Check sheet for the modelled part. Datum: model origin and axes. Units: mm. A direction names the side the tool comes from. Round coordinates to 2 decimals unless told otherwise and drop trailing zeros. Write each loop counter-clockwise with the first axis right and the second up, starting at its lowest first coordinate (ties: lowest second). Pieces come first, ordered by that corner, then holes. Notation, with made-up numbers: (-23.5, 10.25) -> (-2.5, 10.25) arc R27 ccw to (-2.5, 32.25) -> close; hole circle Ø11 at (53, 35). An arc over 180 degrees is marked (long way). Put each result on its own line as item: value. Start each with the question number.
from build123d import *

# Parameters (mm, degrees)
F0_R     = 19.05
F0_R_2   = 16.51
F0_R_3   = 7.62
F0_R_4   = 4.8407005088
F1_DEPTH = 5
F2_START = 5
F0_R_5   = 2.25
F2_DEPTH = 10
F3_START = 12
F3_DEPTH = 8


with BuildPart() as f1:
    # F0 (on Top) → F1 (new body)
    with BuildSketch(Plane.XY):
        Circle(F0_R)
        Circle(F0_R_2, mode=Mode.SUBTRACT)
        Circle(F0_R_2)
        Circle(F0_R_3, mode=Mode.SUBTRACT)
        Circle(F0_R_3)
        Circle(F0_R_4, mode=Mode.SUBTRACT)
    extrude(amount=F1_DEPTH)

    # F0 (on Top) → F2 (join)
    with BuildSketch(Plane.XY.offset(F2_START)):
        Circle(F0_R)
        Circle(F0_R_2, mode=Mode.SUBTRACT)
        Circle(F0_R_3)
        Circle(F0_R_4, mode=Mode.SUBTRACT)
        Circle(F0_R_4)
        Polygon((-2.865183893, 3.6227137055), (1.7047701531, 4.2926788907), (4.5699540462, 0.6699651851), (2.865183893, -3.6227137055), (-1.7047701531, -4.2926788907), (-4.5699540462, -0.6699651851), align=None, mode=Mode.SUBTRACT)
        Polygon((4.5699540462, 0.6699651851), (1.7047701531, 4.2926788907), (-2.865183893, 3.6227137055), (-4.5699540462, -0.6699651851), (-1.7047701531, -4.2926788907), (2.865183893, -3.6227137055), align=None)
        Circle(F0_R_5, mode=Mode.SUBTRACT)
    extrude(amount=F2_DEPTH)

    # F0 (on Top) → F3 (cut)
    with BuildSketch(Plane.XY.offset(F3_START)):
        Polygon((4.5699540462, 0.6699651851), (1.7047701531, 4.2926788907), (-2.865183893, 3.6227137055), (-4.5699540462, -0.6699651851), (-1.7047701531, -4.2926788907), (2.865183893, -3.6227137055), align=None)
        Circle(F0_R_5, mode=Mode.SUBTRACT)
    extrude(amount=F3_DEPTH, mode=Mode.SUBTRACT)


solid = f1.part
1. Section check A-A, the plane z = 13.25. Enter the section's corners in (x, y).
2. Material ranges on L1, parallel to Y at x = 0, z = 10; L2, parallel to X at y = 5, z = 9.75; L3, parallel to X at y = -4.5, z = 9.25, recorded low to high. Write a range as [from, to].
3. Section check D-D, the plane z = 6.75. Enter the section's corners in (x, y).
4. Section check C-C, the plane x = 0. Enter the section's corners in (y, z).
5. Gauge pin test, flat ends, axial feed: P1, Ø4.5, axis at x = -1.5, y = 0, coming from the +Z side; P2, Ø6, axis at x = 0, y = 0, coming from the -Z side; P3, Ø1, axis at x = 0.5, y = -9.5, coming from the +Z side. Record the tip position at first contact, or that the pin passes through.
6. Draft check along Y on faces 1 (the cylindrical face through (-15.12, -11.59, 7.4)), 2 (the flat face through (-6, 16, 15)), 3 (the flat face through (-0.548, 3.962, 13.479)), 4 (the cylindrical face through (4.62, 1.45, 2.46)). Enter one of: released by +Y, released by -Y, zero draft, split by the parting line, or undercut.
7. Section check B-B, the plane y = 14. Enter the section's corners in (x, z), then the cut area to 3 significant figures.
8. Access from +Z, -Z, +X, -X, +Y, -Y to the whole of each face (thin tool, end or side, straight path). Record for faces 5 (the flat face through (3.3, -3.3, 15)), 6 (the flat face through (-2, -2, 12)), 7 (the flat face through (-2.2, -1, 5)).
Reply:
1. outline: circle Ø38.1 at (0, 0); circle Ø15.24 at (0, 0); hole circle Ø33.02 at (0, 0); hole (-4.57, -0.67) -> (-1.7, -4.29) -> (2.87, -3.62) -> (4.57, 0.67) -> (1.7, 4.29) -> (-2.87, 3.62) -> close
2. L1: y = [-19.05, -16.51], [-7.62, -2.25], [2.25, 7.62], [16.51, 19.05]
2. L2: x = [-18.38, -15.73], [-5.75, 5.75], [15.73, 18.38]
2. L3: x = [-18.51, -15.88], [-6.15, 6.15], [15.88, 18.51]
3. outline: circle Ø38.1 at (0, 0); circle Ø15.24 at (0, 0); hole circle Ø33.02 at (0, 0); hole circle Ø4.5 at (0, 0)
4. outline: (-19.05, 0) -> (-4.84, 0) -> (-4.84, 5) -> (-2.25, 5) -> (-2.25, 12) -> (-4.04, 12) -> (-4.04, 15) -> (-7.62, 15) -> (-7.62, 5) -> (-16.51, 5) -> (-16.51, 15) -> (-19.05, 15) -> close; (2.25, 5) -> (4.84, 5) -> (4.84, 0) -> (19.05, 0) -> (19.05, 15) -> (16.51, 15) -> (16.51, 5) -> (7.62, 5) -> (7.62, 15) -> (4.04, 15) -> (4.04, 12) -> (2.25, 12) -> close
5. P1: stops at z = 12
5. P2: stops at z = 5
5. P3: stops at z = 5
6. face 1: split by the parting line
6. face 2: zero draft
6. face 3: undercut
6. face 4: undercut
7. outline: (-12.92, 0) -> (12.92, 0) -> (12.92, 15) -> (8.75, 15) -> (8.75, 5) -> (-8.75, 5) -> (-8.75, 15) -> (-12.92, 15) -> close
7. area: 213 mm2
8. face 5: +Z, +X, -X, +Y, -Y
8. face 6: +Z
8. face 7: -Z
